Verification items for the finished model (mm, model axes). A direction names the side the tool comes from. Round coordinates to 2 decimals unless told otherwise and drop trailing zeros. Write each loop counter-clockwise with the first axis right and the second up, starting at its lowest first coordinate (ties: lowest second). Pieces come first, ordered by that corner, then holes. Notation, with made-up numbers: (67, 71) - (75, 71) arc R24 cw to (75, 96) - close; hole circle Ø11 at (70.25, 58.5). An arc over 180 degrees is marked (long way). Write each question's results on one line, items separated by ' | '.
```python
from build123d import *

# Parameters (mm, degrees)
SALIENTE_EXTRUIR1_DEPTH = 10
CROQUIS3_R              = 2
CORTAR_EXTRUIR2_DEPTH   = 10
CROQUIS4_R              = 1.1
CORTAR_EXTRUIR3_DEPTH   = 10


with BuildPart() as part:
    # Croquis1 → Saliente-Extruir1 (new body)
    with BuildSketch(Plane.XY):
        Polygon((-36.499720763, 42.6), (0, 0), (0, -10), (7, -10), (7, 0), (-35.5, 49.6), (-44.5, 49.6), (-44.5, 42.6), align=None)
    extrude(amount=SALIENTE_EXTRUIR1_DEPTH)

    # Croquis3 → Cortar-Extruir2 (cut)
    with BuildSketch(Plane(origin=(0, 49.6, 0), x_dir=(1, 0, 0), z_dir=(0, 1, 0))):
        with Locations(Location((-40.5, -5, 0), (0, 0, 270))):
            Circle(CROQUIS3_R)
    extrude(amount=-CORTAR_EXTRUIR2_DEPTH, mode=Mode.SUBTRACT)

    # Croquis4 → Cortar-Extruir3 (cut)
    with BuildSketch(Plane(origin=(7, 0, 0), x_dir=(0, 0, -1), z_dir=(1, 0, 0))):
        with Locations((-5, -5)):
            Circle(CROQUIS4_R)
    extrude(amount=-CORTAR_EXTRUIR3_DEPTH, mode=Mode.SUBTRACT)


solid = part.part
```
(1) Section check B-B (z = 5). Record the cut outline in (x, y), plus the area to 3 significant figures.
Answer:
outline: (-44.5, 42.6) - (-42.5, 42.6) - (-42.5, 49.6) - (-44.5, 49.6) - close; (-38.5, 42.6) - (-36.5, 42.6) - (0, 0) - (0, -3.9) - (7, -3.9) - (7, 0) - (-35.5, 49.6) - (-38.5, 49.6) - close; (0, -10) - (7, -10) - (7, -6.1) - (0, -6.1) - close | area: 409 mm2
(2) Mould release check, pull along Z, two halves, no side actions. Record for faces 1 (the flat face through (-15, 20, 10)), 2 (the flat face through (3, -10, 5)), 3 (the cylindrical face through (3.55, -4.07, 4.41)): released by +Z, released by -Z, zero draft, split by the parting line, or undercut.
Answer:
face 1: released by +Z | face 2: zero draft | face 3: undercut
(3) Section check D-D (z = 9). Record the cut outline in (x, y), plus the area to 3 significant figures.
Answer:
outline: (-44.5, 42.6) - (-36.5, 42.6) - (0, 0) - (0, -10) - (7, -10) - (7, 0) - (-35.5, 49.6) - (-44.5, 49.6) - close | area: 452 mm2
(4) Section check C-C (x = -40.5). Record the cut outline in (y, z).
Answer:
outline: (42.6, 0) - (49.6, 0) - (49.6, 3) - (42.6, 3) - close; (42.6, 7) - (49.6, 7) - (49.6, 10) - (42.6, 10) - close
(5) Section check A-A (y = -5). Record the cut outline in (x, z).
Answer:
outline: (0, 0) - (7, 0) - (7, 3.9) - (0, 3.9) - close; (0, 6.1) - (7, 6.1) - (7, 10) - (0, 10) - close
(6) Go/stop test with flat-tipped pins: pin 1 Ø3 at (y, z) = (38.5, 4.5) entering from +X; pin 2 Ø4 at (x, z) = (-42, 5.5) entering from -Y; pin 3 Ø5 at (y, z) = (-5, 3) entering from -X; pin 4 Ø3.5 at (x, z) = (-40.5, 5) entering from -Y. Record where each tip stops, or that it passes through.
Answer:
pin 1: x = -24.7 | pin 2: y = 42.6 | pin 3: x = 0 | pin 4: through
(7) Set-up check for faces 4 (the flat face through (-38, 49.6, 5)), 5 (the flat face through (-42.3, 42.6, 3.8)): record each of +Z, -Z, +X, -X, +Y, -Y from which the full face is reachable in a straight line by a thin tool's end or side.
Answer:
face 4: +Z, -Z, +X, -X, +Y | face 5: +Z, -Z, -X, -Y
(8) Thickness scan on L1, parallel to X at y = 48.25, z = 5; L2, parallel to Y at x = 4.25, z = 5; L3, parallel to Y at x = 1.5, z = 5. Record the ranges inside material, lowest first.
Answer:
L1: -44.5 to -42.5, -38.5 to -34.34 | L2: -10 to -6.1, -3.9 to 3.21 | L3: -10 to -6.1, -3.9 to 6.42
